Geometry check sheet. Reference: drawing and pictorial views, mm from the part's lowest x, y, z. A direction names the side the tool comes from. Give positions to 0.01 mm unless a question says otherwise; leave off trailing zeros. Order: outer loops, then holes, each group sorted by start corner. A loop starts at its lowest first (then second) coordinate and runs counter-clockwise, first axis right, second up. Notation, with made-up numbers: M 79,-15.5 L 83,-15.5 A24 ccw 83,-0.5 Z; hole C 33,18 d5. An arc over 180 degrees is marked long. Answer as CSV lines item,"result". Start each with the question number.
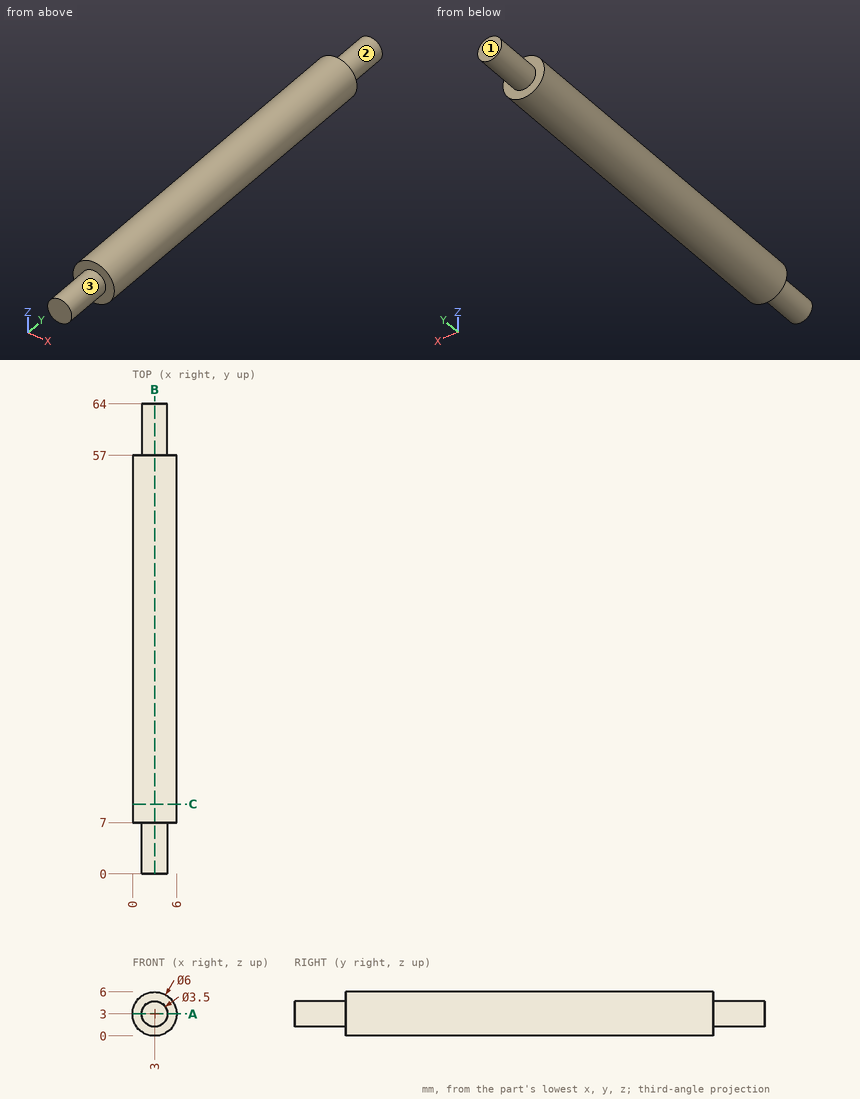
Item 1: Section check A-A on z = 3. Record the boundary of the cut face in (x, y).
Item 2: Scan lines: line 1 along Y through (x, z) = (5, 3.25); line 2 along Z through (x, y) = (3.2, 20). Record each from-to range of solid material in increasing order.
Item 3: Section check C-C on y = 9.5. Record the boundary of the cut face in (x, z).
Item 4: Section check B-B on x = 3. Record the boundary of the cut face in (y, z), then the cut area to 3 significant figures.
Item 5: Access from +Z, -Z, +X, -X, +Y, -Y to the whole of each face (thin tool, end or side, straight path). Record for the marked faces 1, 2 and 3.
Item 6: Depth check by flat-ended pin: pin 1 Ø2 at (x, z) = (5.5, 1) entering from -Y. Enter the tip coordinate at first touch or a pass-through.
Numbers:
1,outline,"M 0,7 L 1.25,7 L 1.25,0 L 4.75,0 L 4.75,7 L 6,7 L 6,57 L 4.75,57 L 4.75,64 L 1.25,64 L 1.25,57 L 0,57 Z"
2,line 1,"7 to 57"
2,line 2,"0.01 to 5.99"
3,outline,"C 3,3 d6"
4,outline,"M 0,1.25 L 7,1.25 L 7,0 L 57,0 L 57,1.25 L 64,1.25 L 64,4.75 L 57,4.75 L 57,6 L 7,6 L 7,4.75 L 0,4.75 Z"
4,area,"349 mm2"
5,face 1,"+Z, -Z, +X, -X, +Y"
5,face 2,"+Y"
5,face 3,"-Y"
6,pin 1,"y = 7"
